from build123d import *

# Parameters (mm, degrees)
MAIN_DEPTH               = 23.75
SKETCH2_R                = 5
SKETCH2_R_2              = 1.25
PLOT_DEPTH               = 3
SKETCH4_R                = 1.25
FIXHOLE_DEPTH            = 11
SKETCH3_W                = 25
SKETCH3_H                = 27.5
CENTRALHOLE_DEPTH        = 11
SKETCH5_R                = 1.5
MAKERBEAMFIXHOLE_DEPTH   = 38
SKETCH6_W                = 35
SKETCH6_H                = 2.9
MAKERBEAMOTHERRAIL_DEPTH = 1
SKETCH7_R                = 1.5
CUT_EXTRUDE4_DEPTH       = 50.5


with BuildPart() as part:
    # Sketch1 → Main (new body, symmetric)
    with BuildSketch(Plane.XY):
        Polygon((-17.5, 5), (-17.5, 1.45), (-18.5, 1.45), (-18.5, -1.45), (-17.5, -1.45), (-17.5, -5), (17.5, -5), (17.5, -1.45), (18.5, -1.45), (18.5, 1.45), (17.5, 1.45), (17.5, 5), align=None)
    extrude(amount=MAIN_DEPTH, both=True)

    # Sketch2 → Plot (add)
    with BuildSketch(Plane(origin=(0, 5, 0), x_dir=(1, 0, 0), z_dir=(0, 1, 0))):
        with Locations((-11.25, 18.75)):
            Circle(SKETCH2_R)
        with Locations((-11.25, 18.75)):
            Circle(SKETCH2_R_2, mode=Mode.SUBTRACT)
        with Locations((-11.25, -18.75)):
            Circle(SKETCH2_R)
        with Locations((-11.25, -18.75)):
            Circle(SKETCH2_R_2, mode=Mode.SUBTRACT)
        with Locations((11.25, 18.75)):
            Circle(SKETCH2_R)
        with Locations((11.25, 18.75)):
            Circle(SKETCH2_R_2, mode=Mode.SUBTRACT)
        with Locations((11.25, -18.75)):
            Circle(SKETCH2_R)
        with Locations((11.25, -18.75)):
            Circle(SKETCH2_R_2, mode=Mode.SUBTRACT)
    extrude(amount=PLOT_DEPTH)

    # Sketch4 → FixHole (cut, through all)
    with BuildSketch(Plane(origin=(0, 5, 0), x_dir=(1, 0, 0), z_dir=(0, 1, 0))):
        with Locations((-11.25, 18.75)):
            Circle(SKETCH4_R)
        with Locations((11.25, 18.75)):
            Circle(SKETCH4_R)
        with Locations((11.25, -18.75)):
            Circle(SKETCH4_R)
        with Locations((-11.25, -18.75)):
            Circle(SKETCH4_R)
    extrude(amount=-FIXHOLE_DEPTH, mode=Mode.SUBTRACT)

    # Sketch3 → CentralHole (cut, through all)
    with BuildSketch(Plane(origin=(0, 5, 0), x_dir=(1, 0, 0), z_dir=(0, 1, 0))):
        Rectangle(SKETCH3_W, SKETCH3_H)
    extrude(amount=-CENTRALHOLE_DEPTH, mode=Mode.SUBTRACT)

    # Sketch5 → MakerBeamFixHole (cut, through all)
    with BuildSketch(Plane.ZY.offset(18.5)):
        Circle(SKETCH5_R)
    extrude(amount=-MAKERBEAMFIXHOLE_DEPTH, mode=Mode.SUBTRACT)

    # Sketch6 → MakerBeamOtherRail (add)
    with BuildSketch(Plane.XY.offset(23.75)):
        Rectangle(SKETCH6_W, SKETCH6_H)
    makerbeamotherrail = extrude(amount=MAKERBEAMOTHERRAIL_DEPTH)

    # Mirror5: MakerBeamOtherRail across plane
    add(makerbeamotherrail.mirror(Plane.XY))

    # Sketch7 → Cut-Extrude4 (cut, through all)
    with BuildSketch(Plane.XY.offset(24.75)):
        Circle(SKETCH7_R)
    extrude(amount=-CUT_EXTRUDE4_DEPTH, mode=Mode.SUBTRACT)


solid = part.part
The model under review builds one solid part; all positions refer to its coordinate system, in mm. A direction names the side the tool comes from. Coordinates: 2 decimals unless noted, no trailing zeros. Loops run counter-clockwise (first coordinate to the right, second up) from the corner with the lowest first, then second, coordinate; pieces in that order, holes last. Notation, with made-up numbers: M 63,72.25 L 93,72.25 A14 cw 93,84.25 Z; hole C 4,-7.5 d3. An arc over 180 degrees is marked long. Put each result on its own line as item: value. Start each with the question number.
Q1. Add section A-A (z = -18.75). Count the separate pieces of the cut face and the enclosed holes in it, and give its area (3 significant figures).
Q2. For faces 1 (the flat face through (-18, 1.45, -12)), 2 (the flat face through (0, -3, -23.75)), 3 (the cylindrical face through (13.557, 6.479, 23.186)), 4 (the flat face through (0, 2, 13.75)), 5 (the flat face through (17.5, 3, 0)), list the 3-axis set-ups (+Z, -Z, +X, -X, +Y, -Y) from which the entire face can be reached by the end or side of a thin tool; tool diameter is ignored.
Q3. Add section C-C (y = -3.5). Write out the cut boundary in (x, z), and give its area (3 significant figures).
Q4. Add section D-D (x = 4). Write out the cut boundary in (y, z).
Q5. Clearance check with flat-ended pins moving along their axes: pin 1 (3 mm diameter, centred on x = -8.5, y = 4, fed in from +Z); pin 2 (1.1 mm diameter, centred on x = 18, z = 6.5, fed in from -Y); pin 3 (1.8 mm diameter, centred on x = -5.5, y = -4, fed in from -Z); pin 4 (5 mm diameter, centred on y = 4, z = 6.5, fed in from -X). State where each tip first meets the part, or that it passes through.
Q6. Add section B-B (z = -11.5). Write out the cut boundary in (x, y).
Q7. Wall thickness on line 1 (Z direction, x = 11.25, y = 1.5); line 2 (X direction, y = 2.5, z = 18.75); line 3 (Z direction, x = 2.5, y = -2.5): over which ranges is each line inside the solid? List them lowest first.
Answers:
1. separate pieces: 3
1. enclosed holes: 1
1. area: 344 mm^2
2. face 1: +Z, -Z, -X, +Y
2. face 2: -Z, +X, -X, -Y
2. face 3: +Y
2. face 4: +Y, -Y
2. face 5: +Z, -Z, +X, +Y
3. outline: M -17.5,-23.75 L 17.5,-23.75 L 17.5,23.75 L -17.5,23.75 Z; hole C -11.25,-18.75 d2.5; hole M -12.5,-13.75 L 12.5,-13.75 L 12.5,13.75 L -12.5,13.75 Z; hole C -11.25,18.75 d2.5; hole C 11.25,-18.75 d2.5; hole C 11.25,18.75 d2.5
3. area: 955 mm^2
4. outline: M -5,-23.75 L -1.45,-23.75 L -1.45,-24.75 L 1.45,-24.75 L 1.45,-23.75 L 5,-23.75 L 5,-13.75 L -5,-13.75 Z; M -5,13.75 L 5,13.75 L 5,23.75 L 1.45,23.75 L 1.45,24.75 L -1.45,24.75 L -1.45,23.75 L -5,23.75 Z
5. pin 1: stops at z = 23.75
5. pin 2: stops at y = -5
5. pin 3: stops at z = -23.75
5. pin 4: stops at x = -17.5
6. outline: M -18.5,-1.45 L -17.5,-1.45 L -17.5,-5 L -12.5,-5 L -12.5,5 L -17.5,5 L -17.5,1.45 L -18.5,1.45 Z; M 12.5,-5 L 17.5,-5 L 17.5,-1.45 L 18.5,-1.45 L 18.5,1.45 L 17.5,1.45 L 17.5,5 L 12.5,5 Z
7. line 1: z = -23.75 to -20, -17.5 to -13.75, 13.75 to 17.5, 20 to 23.75
7. line 2: x = -17.5 to -12.5, -10 to 10, 12.5 to 17.5
7. line 3: z = -23.75 to -13.75, 13.75 to 23.75
